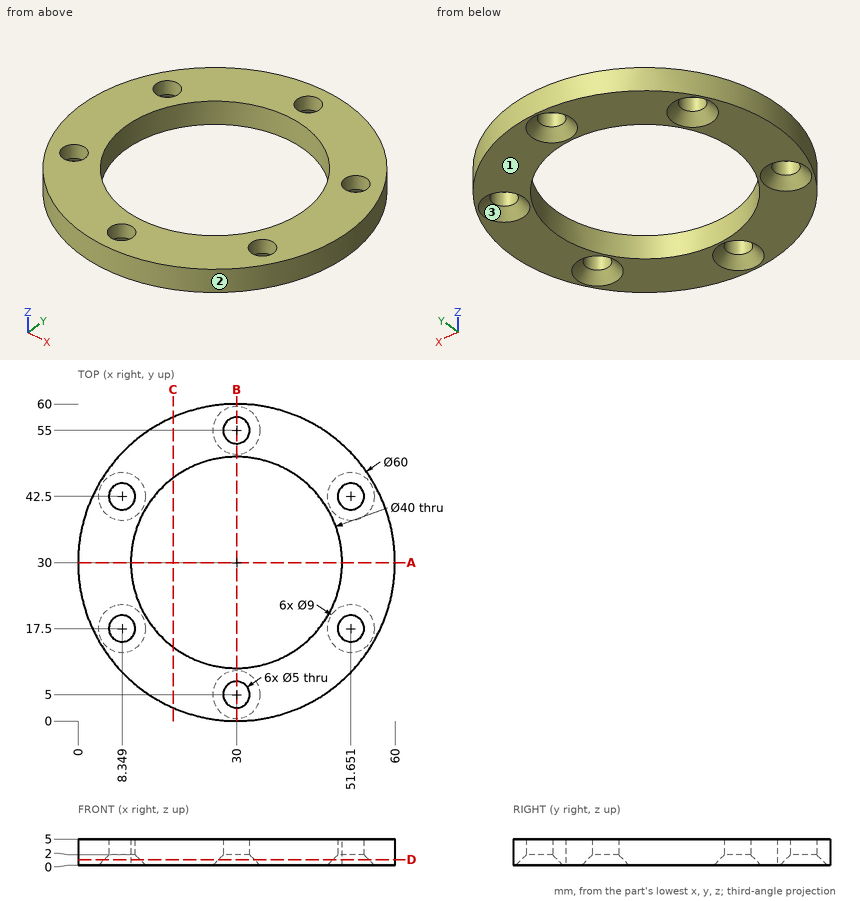
Geometry check sheet. Reference: drawing and pictorial views, mm from the part's lowest x, y, z. Give positions to 0.01 mm unless a question says otherwise; leave off trailing zeros. Order: outer loops, then holes, each group sorted by start corner. A loop starts at its lowest first (then second) coordinate and runs counter-clockwise, first axis right, second up. Notation, with made-up numbers: (5, 13.5) - (56, 13.5) arc R22 cw to (56, 33.5) - close; hole circle Ø7 at (-20, 37.25). An arc over 180 degrees is marked (long way). Answer as CSV lines item,"result".
1. Mould release check, pull along X, two halves, no side actions. Record for the marked faces 1, 2 and 3: released by +X, released by -X, zero draft, split by the parting line, or undercut.
Result sheet:
face 1,"zero draft"
face 2,"split by the parting line"
face 3,"undercut"
2. Scan lines: probe 1 along Y at (x, z) = (30, 3.35); probe 2 along Y at (x, z) = (28, 4.45) (1 decimal); probe 3 along X at (y, z) = (40, 1.1) (1 decimal). Record each from-to range of solid material in increasing order. Write a range as from..to.
Result sheet:
probe 1,"0..2.5, 7.5..10, 50..52.5, 57.5..60"
probe 2,"0.1..3.5, 6.5..10.1, 49.9..53.5, 56.5..59.9"
probe 3,"1.7..6, 10.7..12.7, 47.3..49.3, 54..58.3"
3. Section check D-D (z = 1.1). Record the boundary of the cut face in (x, y), then the cut area to 3 significant figures.
Result sheet:
outline,"circle Ø60 at (30, 30); hole circle Ø6.8 at (8.35, 17.5); hole circle Ø6.8 at (8.35, 42.5); hole circle Ø40 at (30, 30); hole circle Ø6.8 at (30, 5); hole circle Ø6.8 at (30, 55); hole circle Ø6.8 at (51.65, 17.5); hole circle Ø6.8 at (51.65, 42.5)"
area,"1,350 mm²"
4. Go/stop test with a flat-tipped pin: P1, Ø8, axis at x = 8.35, y = 17.5, coming from the -Z side. Record where the tip stops, or that it passes through.
Result sheet:
P1,"z = 0.5"
5. Section check B-B (x = 30). Record the boundary of the cut face in (y, z), then the cut area to 3 significant figures.
Result sheet:
outline,"(0, 0) - (0.5, 0) - (2.5, 2) - (2.5, 5) - (0, 5) - close; (7.5, 2) - (9.5, 0) - (10, 0) - (10, 5) - (7.5, 5) - close; (50, 0) - (50.5, 0) - (52.5, 2) - (52.5, 5) - (50, 5) - close; (57.5, 2) - (59.5, 0) - (60, 0) - (60, 5) - (57.5, 5) - close"
area,"42.0 mm²"
6. Section check A-A (y = 30). Record the boundary of the cut face in (x, z), then the cut area to 3 significant figures.
Result sheet:
outline,"(0, 0) - (10, 0) - (10, 5) - (0, 5) - close; (50, 0) - (60, 0) - (60, 5) - (50, 5) - close"
area,"100 mm²"
7. Section check C-C (x = 18). Record the boundary of the cut face in (y, z) (1 decimal).
Result sheet:
outline,"(2.5, 0) - (14, 0) - (14, 5) - (2.5, 5) - close; (46, 0) - (57.5, 0) - (57.5, 5) - (46, 5) - close"
